Build history of the part. All positions in model axes, mm. Face numbers are marked on the shaded views. Give positions to 0.01 mm unless a question says otherwise; leave off trailing zeros. Write each loop counter-clockwise with the first axis right and the second up, starting at its lowest first coordinate (ties: lowest second). Pieces come first, ordered by that corner, then holes. Notation, with made-up numbers: (22, -13.5) -> (72, -13.5) arc R19 ccw to (72, 6.5) -> close; hole circle Ø8 at (66, 6.5). An arc over 180 degrees is marked (long way). Put each result on its own line as item: value. Start each with the question number.
Item 1: Flat gauge pins, fed straight in: pin 1 Ø6 at (x, z) = (45.5, 6.5) entering from +Y; pin 2 Ø11 at (y, z) = (0, 0) entering from +X; pin 3 Ø10 at (x, y) = (38, -1.5) entering from +Z. Where does each tip first touch, or does it go through?
Item 2: Slice it at A-A, the plane z = 0. List the corners of the cut face in (x, y), plus the area to 3 significant figures.
Item 3: Slice it at D-D, the plane z = -7.5. List the corners of the cut face in (x, y), plus the area to 3 significant figures.
Item 4: Slice it at B-B, the plane y = 6.25. List the corners of the cut face in (x, z).
Item 5: Slice it at C-C, the plane x = 102.5. List the corners of the cut face in (y, z).
Item 6: Drill centre lines: line 1 along Y through (x, z) = (93, 0); line 2 along X through (y, z) = (-1.5, -7); line 3 along Y through (x, z) = (115, -1.25). Where is each one in solid material? Low to high.
Item 7: Two-plate mould, pull along Y, no slides. Class the marked faces 1, 2 and 3: pulls with the +Y half, pulls with the -Y half, needs draft (parallel to the pull), parting line crosses it, or undercut.
Autodesk Fusion 360 part; units mm, degrees
sketch "Esboço1" plane through (0, 0, 0) normal (1, 0, 0) x (0, 1, 0)
  circle A0 centre (0, 0) radius 11.75
  dimension "d1" = 23.5
extrude "Extrusão1" add sketch "Esboço1" along normal blind 120
sketch "Esboço2" plane through (120, 0, 0) normal (1, 0, 0) x (0, 1, 0)
  circle A0 centre (0, 0) radius 11.75
sketch "Esboço3" plane through (120, 0, 0) normal (1, 0, 0) x (0, 1, 0)
  line L0 (-10, 6) -> (-8.3006, 3.7257)
  line L1 (11.1508, 3.7257) -> (8.8709, 2.0221)
  arc A0 (-8.3006, 3.7257) -> (8.8709, 2.0221) centre (0, 0) ccw
  line L2 (-10.8021, 6.8786) -> (-10, 6)
  line L3 (11.8471, 4.8629) -> (11.1508, 3.7257)
  arc A1 (11.8471, 4.8629) -> (-10.8021, 6.8786) centre (0, 0) ccw
  arc A2 (-10.062, 6.0679) -> (11.1451, 3.7214) centre (0, 0) ccw
  dimension "d4" = 23.5
extrude "Extrusão2" cut sketch "Esboço3" against normal blind 105 contours L0 L1 A0 L2 L3 A1
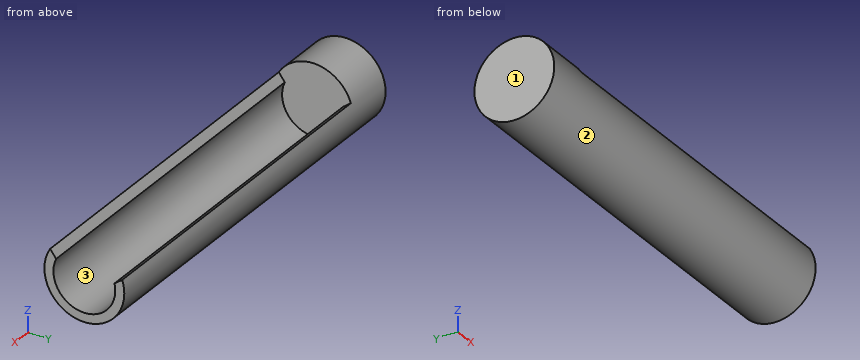
Values follow:
1. pin 1: y = 11.22
1. pin 2: x = 15
1. pin 3: z = -6.37
2. outline: (0, -11.75) -> (120, -11.75) -> (120, -9.1) -> (15, -9.1) -> (15, 9.1) -> (120, 9.1) -> (120, 11.75) -> (0, 11.75) -> close
2. area: 909 mm2
3. outline: (0, -9.05) -> (120, -9.05) -> (120, -5.15) -> (15, -5.15) -> (15, 5.15) -> (120, 5.15) -> (120, 9.05) -> (0, 9.05) -> close
3. area: 1,090 mm2
4. outline: (0, -9.95) -> (120, -9.95) -> (120, -6.61) -> (15, -6.61) -> (15, 9.95) -> (0, 9.95) -> close
5. outline: (-10.06, 6.07) arc R11.75 ccw (long way) to (11.15, 3.72) -> (8.87, 2.02) arc R9.1 cw (long way) to (-8.3, 3.73) -> (-10, 6) -> close
6. line 1: -11.75 to -9.1, 9.1 to 11.75
6. line 2: 0 to 15
6. line 3: -11.68 to -9.01, 9.01 to 11.68
7. face 1: needs draft
7. face 2: parting line crosses it
7. face 3: undercut
